Read the model definition and answer for the solid it produces. Units are mm, in the model's axes. Face numbers are marked on the shaded views. A direction names the side the tool comes from. Coordinates: 2 decimals unless noted, no trailing zeros. Order: outer loops, then holes, each group sorted by start corner. A loop starts at its lowest first (then second) coordinate and runs counter-clockwise, first axis right, second up.
```python
from build123d import *

# Parameters (mm, degrees)
F1_DEPTH = 63.5
F2_DEPTH = 25.4
F3_DEPTH = 7.9375
F5_R     = 6.35


with BuildPart() as f1:
    # F0 (on Front) → F1 (new body, symmetric)
    with BuildSketch(Plane.XZ):
        Polygon((-41.275, 9.525), (-41.275, -9.525), (41.275, -9.525), (41.275, 9.525), (22.225, 9.525), align=None)
    extrude(amount=F1_DEPTH, both=True)

    # F0 (on Front) → F2 (join, symmetric)
    with BuildSketch(Plane.XZ):
        with BuildLine():
            Line((22.225, 9.525), (41.275, 9.525))
            Line((41.275, 9.525), (41.275, 27.0002))
            ThreePointArc((41.275, 27.0002), (45.92468, 38.22552), (57.15, 42.8752))
            Line((57.15, 42.8752), (60.325, 42.8752))
            Line((60.325, 42.8752), (60.325, 61.9252))
            Line((60.325, 61.9252), (57.15, 61.9252))
            ThreePointArc((57.15, 61.9252), (32.454296, 51.695904), (22.225, 27.0002))
            Line((22.225, 27.0002), (22.225, 9.525))
        make_face()
        Polygon((60.325, 66.675), (60.325, 61.9252), (60.325, 42.8752), (60.325, 38.1), (111.125, 38.1), (111.125, 66.675), align=None)
    extrude(amount=F2_DEPTH, both=True)

    # F0 (on Front) → F3 (join, symmetric)
    with BuildSketch(Plane.XZ):
        with BuildLine():
            add(Edge.make_bspline(
                [(-41.275, 9.525), (-21.197749, 53.768482), (17.248105, 69.648288), (57.15, 61.9252)],
                knots=[0, 0, 0, 0, 111.504536, 111.504536, 111.504536, 111.504536], degree=3))
            Line((-41.275, 9.525), (22.225, 9.525))
            Line((22.225, 9.525), (22.225, 27.0002))
            ThreePointArc((22.225, 27.0002), (32.454296, 51.695904), (57.15, 61.9252))
        make_face()
    extrude(amount=F3_DEPTH, both=True)

    # F0 (on Front) → F4 (revolve)
    with BuildSketch(Plane.XZ):
        Polygon((60.325, 66.675), (60.325, 61.9252), (60.325, 42.8752), (60.325, 38.1), (111.125, 38.1), (111.125, 66.675), align=None)
    revolve(axis=Axis((111.125, 0, 52.3875), (0, 0, 1)))

    # F5
    f5_edges = [f1.edges().sort_by_distance(p)[0] for p in [
        (-41.275, -63.5, 0),
        (-41.275, 63.5, 0),
        (41.275, 63.5, 0),
        (41.275, -63.5, 0),
    ]]
    fillet(f5_edges, radius=F5_R)


solid = f1.part
```
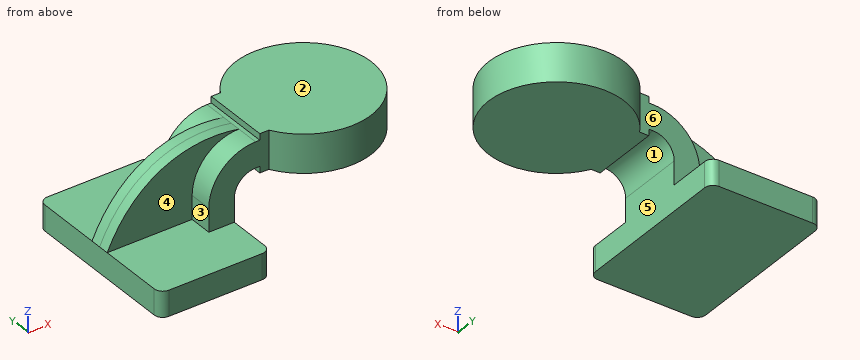
1) Which of the six approach directions +Z, -Z, +X, -X, +Y, -Y give full straight-line access (tool end or side, diameter ignored) to the marked faces 4, 5 and 6?
A:
face 4: +Z, -X, -Y
face 5: -Z, +X, +Y, -Y
face 6: +Z, -X, +Y
2) A cutting plane is placed at D-D, the plane y = -53.5. Determine the outline of the cut face in (x, z) (3 decimals).
A:
outline: (-41.275, -9.525) - (41.275, -9.525) - (41.275, 9.525) - (-41.275, 9.525) - close
3) Straight lines are drawn through the part: line 1 (Y direction, x = -5.5, z = 35); line 2 (X direction, y = -36.5, z = 8) (3 decimals); line 3 (Y direction, x = 61.5, z = 56). For each, find the intervals that lie inside material, in ascending order.
A:
line 1: y = -7.94 to 7.94
line 2: x = -41.275 to 41.275
line 3: y = -25.4 to 25.4
4) A cutting plane is placed at B-B, the plane y = 16.5. Determine the outline of the cut face in (x, z) (3 decimals), and give its area (3 significant figures).
A:
outline: (-41.275, -9.525) - (41.275, -9.525) - (41.275, 27) arc R15.875 cw to (57.15, 42.875) - (60.325, 42.875) - (60.325, 38.1) - (159.171, 38.1) - (159.171, 66.675) - (60.325, 66.675) - (60.325, 61.925) - (57.15, 61.925) arc R34.925 ccw to (22.225, 27) - (22.225, 9.525) - (-41.275, 9.525) - close
area: 5,550 mm2
5) Flat-ended cylindrical pins translate along their axes: pin 1 Ø1 at (x, y) = (59, -12.5) entering from +Z; pin 2 Ø1.4 at (y, z) = (3, 65) entering from -X (3 decimals); pin 3 Ø2.5 at (y, z) = (-6.5, 41) entering from -X; pin 4 Ø8 at (x, z) = (-15, 55) entering from +Y. Find the tip coordinate at first contact, or state that the pin passes through.
A:
pin 1: stops at z = 61.93
pin 2: stops at x = 60.325
pin 3: stops at x = -20.84
pin 4: passes through
6) A cutting plane is placed at A-A, the plane y = 33. Determine the outline of the cut face in (x, z) (3 decimals), and give its area (3 significant figures).
A:
outline: (-41.275, -9.525) - (41.275, -9.525) - (41.275, 9.525) - (-41.275, 9.525) - close; (72.503, 38.1) - (149.747, 38.1) - (149.747, 66.675) - (72.503, 66.675) - close
area: 3,780 mm2
7) A cutting plane is placed at C-C, the plane x = 136.5. Determine the outline of the cut face in (y, z) (3 decimals), and give its area (3 significant figures).
A:
outline: (-44.009, 38.1) - (44.009, 38.1) - (44.009, 66.675) - (-44.009, 66.675) - close
area: 2,520 mm2
8) Determine the mould class of the marked faces 1, 2 and 3 for opening direction X: pulls with the +X half, pulls with the -X half, needs draft (parallel to the pull), parting line crosses it, or undercut.
A:
face 1: undercut
face 2: needs draft
face 3: pulls with the -X half
